from build123d import *

# Parameters (mm, degrees)
SKETCH1_W      = 125
SKETCH1_H      = 290
SKETCH1_R      = 15.5
EXTRUDE1_DEPTH = 12
SKETCH2_W      = 12
SKETCH2_H      = 290
EXTRUDE2_DEPTH = 188
SKETCH3_R      = 15.5
EXTRUDE3_DEPTH = 188


with BuildPart() as part:
    # Sketch1 → Extrude1 (new body)
    with BuildSketch(Plane.XY):
        with Locations((62.5, 145)):
            Rectangle(SKETCH1_W, SKETCH1_H)
        with Locations((41, 45)):
            Circle(SKETCH1_R, mode=Mode.SUBTRACT)
        with Locations((41, 145)):
            Circle(SKETCH1_R, mode=Mode.SUBTRACT)
        with Locations((41, 245)):
            Circle(SKETCH1_R, mode=Mode.SUBTRACT)
    extrude(amount=EXTRUDE1_DEPTH)

    # Sketch2 → Extrude2 (add)
    with BuildSketch(Plane.XY.offset(12)):
        with Locations((119, 145)):
            Rectangle(SKETCH2_W, SKETCH2_H)
    extrude(amount=EXTRUDE2_DEPTH)

    # Sketch3 → Extrude3 (cut)
    with BuildSketch(Plane.ZY.offset(-113)):
        with Locations(Location((159, 45, 0), (0, 0, 270))):
            Circle(SKETCH3_R)
        with Locations(Location((159, 145, 0), (0, 0, 270))):
            Circle(SKETCH3_R)
        with Locations(Location((159, 245, 0), (0, 0, 270))):
            Circle(SKETCH3_R)
        with Locations(Location((79, 95, 0), (0, 0, 270))):
            Circle(SKETCH3_R)
        with Locations(Location((79, 195, 0), (0, 0, 270))):
            Circle(SKETCH3_R)
    extrude(amount=-EXTRUDE3_DEPTH, mode=Mode.SUBTRACT)


solid = part.part
Work out the finished part from the listing and answer in its coordinate system (mm). A direction names the side the tool comes from. Give positions to 0.01 mm unless a question says otherwise; leave off trailing zeros. Loops run counter-clockwise (first coordinate to the right, second up) from the corner with the lowest first, then second, coordinate; pieces in that order, holes last. Notation, with made-up numbers: M 75.25,13.5 L 122.25,13.5 A31 cw 122.25,44.5 Z; hole C 80,24 d2. An arc over 180 degrees is marked long. Use CSV: the item, a comma, the result in double quotes.
1) Find section C-C on z = 79. Write down the section's boundary in (x, y).
Answer:
outline,"M 113,0 L 125,0 L 125,79.5 L 113,79.5 Z; M 113,110.5 L 125,110.5 L 125,179.5 L 113,179.5 Z; M 113,210.5 L 125,210.5 L 125,290 L 113,290 Z"
2) Find section D-D on y = 195. Write down the section's boundary in (x, z), plus the area to 3 significant figures.
Answer:
outline,"M 0,0 L 125,0 L 125,63.5 L 113,63.5 L 113,12 L 0,12 Z; M 113,94.5 L 125,94.5 L 125,200 L 113,200 Z"
area,"3,380 mm^2"
3) Which of the six approach directions +Z, -Z, +X, -X, +Y, -Y give full straight-line access (tool end or side, diameter ignored) to faces 1 (the flat face through (68, 147, 12)), 2 (the cylindrical face through (49.33, 58.07, 5.92))?
Answer:
face 1,"+Z, -X, +Y, -Y"
face 2,"+Z, -Z"
4) Given P1, Ø8, axis at x = 26, y = 186.5, coming from the -Z side; P2, Ø1, axis at y = 146.5, z = 25.5, coming from the -X side; P3, Ø2, axis at x = 62.5, y = 78, coming from the +Z side, each flat-ended and moving along its own axis, determine where each tip first touches the part or whether it passes through.
Answer:
P1,"z = 0"
P2,"x = 113"
P3,"z = 12"
5) Find section B-B on x = 41. Write down the section's boundary in (y, z).
Answer:
outline,"M 0,0 L 29.5,0 L 29.5,12 L 0,12 Z; M 60.5,0 L 129.5,0 L 129.5,12 L 60.5,12 Z; M 160.5,0 L 229.5,0 L 229.5,12 L 160.5,12 Z; M 260.5,0 L 290,0 L 290,12 L 260.5,12 Z"
6) Determine the mould class of faces 3 (the flat face through (125, 143, 99)), 4 (the cylindrical face through (118.916, 160.485, 159.682)), 5 (the cylindrical face through (55.784, 149.656, 5.916)) for opening direction X: released by +X, released by -X, zero draft, split by the parting line, or undercut.
Answer:
face 3,"released by +X"
face 4,"zero draft"
face 5,"undercut"
7) Consider L1, parallel to Y at x = 41, z = 5; L2, parallel to Z at x = 115, y = 195; L3, parallel to X at y = 116, z = 131. Determine where each line is inside the solid, lowest interval first.
Answer:
L1,"0 to 29.5, 60.5 to 129.5, 160.5 to 229.5, 260.5 to 290"
L2,"0 to 63.5, 94.5 to 200"
L3,"113 to 125"
8) Find section A-A on y = 45. Write down the section's boundary in (x, z), plus the area to 3 significant figures.
Answer:
outline,"M 0,0 L 25.5,0 L 25.5,12 L 0,12 Z; M 56.5,0 L 125,0 L 125,143.5 L 113,143.5 L 113,12 L 56.5,12 Z; M 113,174.5 L 125,174.5 L 125,200 L 113,200 Z"
area,"3,010 mm^2"
